The model under review builds one solid part; all positions refer to its coordinate system, in mm. Give positions to 0.01 mm unless a question says otherwise; leave off trailing zeros. Write each loop counter-clockwise with the first axis right and the second up, starting at its lowest first coordinate (ties: lowest second). Pieces come first, ordered by that corner, then holes. Notation, with made-up numbers: (26, 63) -> (42, 63) arc R14 cw to (42, 86) -> close; hole circle Ø5 at (84, -36.5). An arc over 180 degrees is marked (long way). Use CSV: the item, a comma, the result in double quotes.
Autodesk Inventor part; units mm, degrees
ref_plane "YZ Plane" through (0, 0, 0) normal (1, 0, 0) x (0, 1, 0)
ref_plane "XZ Plane" through (0, 0, 0) normal (0, 1, 0) x (-1, 0, 0)
ref_plane "XY Plane" through (0, 0, 0) normal (0, 0, 1) x (1, 0, 0)
sketch "Sketch1" plane through (0, 0, 0) normal (1, 0, 0) x (0, 1, 0)
  line L0 (12.1919, 24.5577) -> (-64.8081, 24.5577)
  line L1 (-64.8081, 24.5577) -> (-64.8081, 6.5577)
  line L2 (-64.8081, 6.5577) -> (12.1919, 6.5577)
  line L3 (12.1919, 6.5577) -> (12.1919, 24.5577)
  point P0 (0, 0)
  dimension "d0" = 77
  dimension "d1" = 18
extrude "Plate1" add sketch "Sketch1" along normal blind 6.5
sketch "Sketch2" plane through (0, -64.8081, 24.5577) normal (0, 0, 1) x (1, 0, 0)
  point P0 (0, 64.8081)
  point P1 (3.3009, 71.2411)
hole "Hole1" at (3.3009, 6.4331, 24.5577) direction (0, 0, -1) diameter 6 end through all
equation "\"d8\" = Thickness"
equation "\"d2\" = Thickness"
equation "\"BendRadius\" = Thickness"
equation "\"BendReliefWidth\" = Thickness"
equation "\"BendReliefDepth\" = 0.5 * Thickness"
equation "\"CornerReliefSize\" = 4 * Thickness"
equation "\"MinimumRemnant\" = 2 * Thickness"
equation "\"TransitionRadius\" = BendRadius"
equation "\"JacobiRadiusSize\" = BendRadius"
equation "\"GapSize\" = Thickness"
properties part number "blde"
Q1. To check wall thickness, follow probe 1 along Y at (x, z) = (3.25, 15); probe 2 along Y at (x, z) = (4, 14.5); probe 3 along X at (y, z) = (4.5, 13). State the ranges of each line that lie inside material, in increasing order.
Derived:
probe 1,"y = -64.81 to 3.43, 9.43 to 12.19"
probe 2,"y = -64.81 to 3.52, 9.35 to 12.19"
probe 3,"x = 0 to 1.01, 5.6 to 6.5"
Q2. Consider section C-C (z = 17.5). Write out the cut boundary in (x, y), then the cut area to 3 significant figures.
Derived:
outline,"(0, -64.81) -> (6.5, -64.81) -> (6.5, 12.19) -> (0, 12.19) -> close; hole circle Ø6 at (3.3, 6.43)"
area,"472 mm2"
Q3. Consider section B-B (y = 4.5). Write out the cut boundary in (x, z), then the cut area to 3 significant figures.
Derived:
outline,"(0, 6.56) -> (1.01, 6.56) -> (1.01, 24.56) -> (0, 24.56) -> close; (5.6, 6.56) -> (6.5, 6.56) -> (6.5, 24.56) -> (5.6, 24.56) -> close"
area,"34.4 mm2"
Q4. Consider section A-A (x = 1.75). Write out the cut boundary in (y, z).
Derived:
outline,"(-64.81, 6.56) -> (3.87, 6.56) -> (3.87, 24.56) -> (-64.81, 24.56) -> close; (9, 6.56) -> (12.19, 6.56) -> (12.19, 24.56) -> (9, 24.56) -> close"
